from build123d import *

# Parameters (mm, degrees)
SKETCH1_R           = 1.414036492
SKETCH1_R_2         = 1.5
BOSS_EXTRUDE1_DEPTH = 1.8


with BuildPart() as part:
    # Sketch1 → Boss-Extrude1 (new body)
    with BuildSketch(Plane.XY):
        Polygon((-14.604832392, 9.639595654), (-14.604832392, 6.577460034), (-18.658403667, 6.577460034), (-18.658403667, -14.020338192), (-14.604832392, -14.020338192), (-14.604832392, -21.750404346), (16.995167608, -21.750404346), (16.995167608, -18.750404346), (22.995167608, -18.750404346), (22.995167608, -12.757063543), (16.995167608, -12.750404346), (16.995167608, 19.849595654), (-14.894517711, 19.849595654), (-14.894517711, 15.639595654), (-20.550663677, 15.639595654), (-20.550663677, 9.639595654), align=None)
        with Locations((-17.550663677, 12.639595654)):
            Circle(SKETCH1_R, mode=Mode.SUBTRACT)
        with Locations((19.995167608, -15.753900813)):
            Circle(SKETCH1_R_2, mode=Mode.SUBTRACT)
    extrude(amount=BOSS_EXTRUDE1_DEPTH)


solid = part.part
The listing builds one solid part. Answer for the finished solid, in the listing's coordinates (mm). A direction names the side the tool comes from. Coordinates: 2 decimals unless noted, no trailing zeros. Order: outer loops, then holes, each group sorted by start corner. A loop starts at its lowest first (then second) coordinate and runs counter-clockwise, first axis right, second up. Notation, with made-up numbers: M 38.5,-25 L 58.5,-25 A25 ccw 58.5,-6 Z; hole C 33.5,-23 d3. An arc over 180 degrees is marked long. Use CSV: the item, a comma, the result in double quotes.
Q1. Straight lines are drawn through the part: L1, parallel to Y at x = -18, z = 0.8; L2, parallel to Y at x = 18, z = 0.1; L3, parallel to X at y = -3, z = 0.3. For each, find the intervals that lie inside material, in ascending order.
Here are the results:
L1,"-14.02 to 6.58, 9.64 to 11.3, 13.98 to 15.64"
L2,"-18.75 to -12.75"
L3,"-18.66 to 17"
Q2. A tool of negligible diameter and unlimited length cuts with its end or side. For faces 4 (the flat face through (-14.605, -18, 1)), 5 (the flat face through (-18, 9.64, 1)), 6 (the flat face through (-18, 15.64, 1)), from which of +Z, -Z, +X, -X, +Y, -Y can it reach the whole face along a straight path? Write none if from no direction.
Here are the results:
face 4,"+Z, -Z, -X, -Y"
face 5,"+Z, -Z, -X"
face 6,"+Z, -Z, -X, +Y"
Q3. Section A-A (x = 19.5) is taken. Determine the outline of the cut face in (y, z).
Here are the results:
outline,"M -18.75,0 L -17.17,0 L -17.17,1.8 L -18.75,1.8 Z; M -14.34,0 L -12.75,0 L -12.75,1.8 L -14.34,1.8 Z"
Q4. Section B-B (x = -17) is taken. Determine the outline of the cut face in (y, z).
Here are the results:
outline,"M -14.02,0 L 6.58,0 L 6.58,1.8 L -14.02,1.8 Z; M 9.64,0 L 11.34,0 L 11.34,1.8 L 9.64,1.8 Z; M 13.94,0 L 15.64,0 L 15.64,1.8 L 13.94,1.8 Z"
Q5. Given pin 1 Ø1 at (y, z) = (9.5, 0.5) entering from +X; pin 2 Ø0.5 at (x, z) = (-17, 1) entering from +Y; pin 3 Ø0.5 at (y, z) = (18.5, 0.5) entering from -X, each flat-ended and moving along its own axis, determine where each tip first touches the part or whether it passes through.
Here are the results:
pin 1,"x = 17"
pin 2,"y = 15.64"
pin 3,"x = -14.89"
Q6. Section C-C (y = 12) is taken. Determine the outline of the cut face in (x, z), then the cut area to 3 significant figures.
Here are the results:
outline,"M -20.55,0 L -18.81,0 L -18.81,1.8 L -20.55,1.8 Z; M -16.29,0 L 17,0 L 17,1.8 L -16.29,1.8 Z"
area,"63.0 mm2"
Q7. Determine the mould class of faces 1 (the flat face through (-17, 6.577, 1)), 2 (the cylindrical face through (-16.898, 11.385, 0.887)), 3 (the flat face through (22.995, -16, 1)) for opening direction X: pulls with the +X half, pulls with the -X half, needs draft (parallel to the pull), parting line crosses it, or undercut.
Here are the results:
face 1,"needs draft"
face 2,"undercut"
face 3,"pulls with the +X half"
Q8. Section D-D (z = 1.3) is taken. Determine the outline of the cut face in (x, y).
Here are the results:
outline,"M -20.55,9.64 L -14.6,9.64 L -14.6,6.58 L -18.66,6.58 L -18.66,-14.02 L -14.6,-14.02 L -14.6,-21.75 L 17,-21.75 L 17,-18.75 L 23,-18.75 L 23,-12.76 L 17,-12.75 L 17,19.85 L -14.89,19.85 L -14.89,15.64 L -20.55,15.64 Z; hole C -17.55,12.64 d2.83; hole C 20,-15.75 d3"
